from build123d import *

# Parameters (mm, degrees)
F1_DEPTH = 31.75


with BuildPart() as f1:
    # F0 (on Front) → F1 (new body, symmetric)
    with BuildSketch(Plane.XZ):
        Polygon((5.472675, 0.224179), (2.542193, 4.851565), (-2.930482, 4.627386), (-5.472675, -0.224179), (-2.542193, -4.851565), (2.930482, -4.627386), align=None)
        Polygon((-2.145882, 3.388461), (1.861552, 3.552618), (4.007434, 0.164158), (2.145882, -3.388461), (-1.861552, -3.552618), (-4.007434, -0.164158), align=None, mode=Mode.SUBTRACT)
    extrude(amount=F1_DEPTH, both=True)


solid = f1.part
The listing builds one solid part. Answer for the finished solid, in the listing's coordinates (mm). A direction names the side the tool comes from. Coordinates: 2 decimals unless noted, no trailing zeros. Loops run counter-clockwise (first coordinate to the right, second up) from the corner with the lowest first, then second, coordinate; pieces in that order, holes last.
1) Find the intervals of material crossed by L1, parallel to X at y = 26, z = -1.75; L2, parallel to X at y = -15, z = -0.75; L3, parallel to Z at x = 0.5, y = -5, in increasing order.
2) Find section A-A on y = 21. Write down the section's boundary in (x, z), then the cut area to 3 significant figures.
3) Flat-ended cylindrical pins translate along their axes: pin 1 Ø5 at (x, y) = (-1.5, -2.5) entering from -Z; pin 2 Ø5 at (y, z) = (-12.5, -1) entering from -X; pin 3 Ø1.5 at (x, y) = (-2.5, -1.5) entering from +Z; pin 4 Ø3 at (x, y) = (3, -19) entering from -Z. Find the tip coordinate at first contact, or state that the pin passes through.
4) Find section C-C on x = 0.75. Write down the section's boundary in (y, z), then the cut area to 3 significant figures.
5) A tool of negligible diameter and unlimited length cuts with its end or side. For faces 1 (the face through (-3.09, -0.44, 1.59)), 2 (the face through (0, -31.75, -4)), from which of +Z, -Z, +X, -X, +Y, -Y can it reach the whole face along a straight path? Write none if from no direction.
6) Determine the mould class of faces 3 (the face through (-0.17, -0.44, 3.47)), 4 (the face through (-4.18, -0.44, 2.24)), 5 (the face through (4.028, -0.444, 2.505)) for opening direction X: pulls with the +X half, pulls with the -X half, needs draft (parallel to the pull), parting line crosses it, or undercut.
7) Find section B-B on z = -2.5. Write down the section's boundary in (x, y).
Values:
1. L1: x = -4.51 to -3, 3 to 4.44
1. L2: x = -5.14 to -3.64, 3.53 to 4.96
1. L3: z = -4.73 to -3.46, 3.5 to 4.77
2. outline: (-5.47, -0.22) - (-2.54, -4.85) - (2.93, -4.63) - (5.47, 0.22) - (2.54, 4.85) - (-2.93, 4.63) - close; hole (-4.01, -0.16) - (-1.86, -3.55) - (2.15, -3.39) - (4.01, 0.16) - (1.86, 3.55) - (-2.15, 3.39) - close
2. area: 36.1 mm2
3. pin 1: stops at z = -4.85
3. pin 2: stops at x = -5.47
3. pin 3: stops at z = 4.68
3. pin 4: stops at z = -4.69
4. outline: (-31.75, -4.72) - (31.75, -4.72) - (31.75, -3.45) - (-31.75, -3.45) - close; (-31.75, 3.51) - (31.75, 3.51) - (31.75, 4.78) - (-31.75, 4.78) - close
4. area: 161 mm2
5. face 1: +Y, -Y
5. face 2: +Z, -Z, +X, -X, -Y
6. face 3: undercut
6. face 4: pulls with the -X half
6. face 5: pulls with the +X half
7. outline: (-4.03, -31.75) - (-2.53, -31.75) - (-2.53, 31.75) - (-4.03, 31.75) - close; (2.61, -31.75) - (4.05, -31.75) - (4.05, 31.75) - (2.61, 31.75) - close
